Autodesk Inventor part; units mm, degrees
ref_plane "YZ Plane" through (0, 0, 0) normal (1, 0, 0) x (0, 1, 0)
ref_plane "XZ Plane" through (0, 0, 0) normal (0, 1, 0) x (-1, 0, 0)
ref_plane "XY Plane" through (0, 0, 0) normal (0, 0, 1) x (1, 0, 0)
sketch "Boceto1" plane through (0, 0, 0) normal (0, 0, 1) x (1, 0, 0)
  line L0 (-45, 21.0335) -> (-45, 0)
  line L1 (-43.1, 4) -> (-1.9, 4)
  line L2 (0, 0) -> (0, 15.6)
  line L3 (-4.7, 44) -> (-4.7, 21.3767)
  line L4 (-4.7, 44) -> (-9.9, 44)
  line L5 (-8.5, 42.6) -> (-6.1, 42.6)
  line L6 (-6.1, 36.1) -> (-8.5, 36.1)
  line L7 (-43.6, 19.6) -> (-5.4, 19.6)
  line L8 (-1.4, 15.6) -> (-1.4, 5.9)
  line L9 (-1.9, 5.4) -> (-43.1, 5.4)
  line L10 (-43.6, 5.9) -> (-43.6, 19.6)
  arc A0 (0, 15.6) -> (-4.3017, 20.8871) centre (-5.4, 15.6) ccw
  arc A1 (-1.4, 15.6) -> (-5.4, 19.6) centre (-5.4, 15.6) ccw
  line L11 (-1.4, 3.5) -> (-1.4, 1.7468)
  line L12 (-2.5, 0) -> (0, 0)
  line L13 (-6.1, 21.5) -> (-6.1, 34.7)
  line L14 (-6.1, 36.1) -> (-6.1, 42.6)
  line L15 (-43.6, 3.5) -> (-43.6, 1.6777)
  line L16 (-42.5, 0) -> (-45, 0)
  line L17 (-42.5, 0) -> (-42.5, 0.4554)
  line L18 (-2.5, 0) -> (-2.5, 0.7)
  line L19 (-43.6, 21) -> (-43.6, 24)
  line L20 (-42.48, 25.4) -> (-45, 25.4)
  line L21 (-45, 25.4) -> (-45, 21.0335)
  line L22 (-24, 21) -> (-24, 25.4)
  line L23 (-24, 25.4) -> (-26.39, 25.4)
  line L24 (-25.4, 24) -> (-25.4, 21)
  line L25 (-6.6, 21) -> (-24, 21)
  line L26 (-25.4, 21) -> (-43.6, 21)
  line L27 (-41.6, 24) -> (-43.6, 24)
  line L28 (-27.4, 24) -> (-25.4, 24)
  line L29 (-42.7447, 0.8853) -> (-43.3553, 1.2478)
  line L30 (-2.5, 0.7) -> (-1.6082, 1.3408)
  line L31 (-41.6, 24) -> (-41.6, 24.695)
  line L32 (-27.4, 24) -> (-27.4, 24.7058)
  line L33 (-42.48, 25.4) -> (-41.6, 24.695)
  line L34 (-27.4, 24.7058) -> (-26.39, 25.4)
  line L35 (-6.1, 34.7) -> (-9.9, 34.7)
  line L36 (-8.5, 37.35) -> (-8.5, 36.1)
  line L37 (-8.5, 41.35) -> (-8.5, 42.6)
  line L38 (-8.5, 37.35) -> (-9.2058, 37.35)
  line L39 (-8.5, 41.35) -> (-9.2058, 41.35)
  line L40 (-9.9, 44) -> (-9.9, 42.36)
  line L41 (-9.9, 42.36) -> (-9.2058, 41.35)
  line L42 (-9.9, 34.7) -> (-9.9, 36.34)
  line L43 (-9.9, 36.34) -> (-9.2058, 37.35)
  arc A2 (-6.6, 21) -> (-6.1, 21.5) centre (-6.6, 21.5) ccw
  arc A3 (-4.7, 21.3767) -> (-4.3017, 20.8871) centre (-4.2, 21.3767) ccw
  arc A4 (-1.9, 5.4) -> (-1.4, 5.9) centre (-1.9, 5.9) ccw
  arc A5 (-1.4, 3.5) -> (-1.9, 4) centre (-1.9, 3.5) ccw
  arc A6 (-1.6082, 1.3408) -> (-1.4, 1.7468) centre (-1.9, 1.7468) ccw
  arc A7 (-43.6, 5.9) -> (-43.1, 5.4) centre (-43.1, 5.9) ccw
  arc A8 (-43.1, 4) -> (-43.6, 3.5) centre (-43.1, 3.5) ccw
  arc A9 (-43.6, 1.6777) -> (-43.3553, 1.2478) centre (-43.1, 1.6777) ccw
  line L44 (0, 4) -> (0, 4.0335)
  arc A10 (-42.5, 0.4554) -> (-42.7447, 0.8853) centre (-43, 0.4554) ccw
  point P0 (-8.5, 41.975)
  point P1 (-42.5, 4)
  point P2 (-6.1, 39.35)
  point P3 (-42.5, 0.74)
  dimension "d16" = 5.4
  dimension "d17" = 4
  dimension "d32" = 1.4
  dimension "d35" = 1.4
  dimension "d37" = 3
  dimension "d38" = 25.4
  dimension "d44" = 18.2
  dimension "d50" = 0.7
  dimension "d53" = 40.3
  dimension "d54" = 37.5
  dimension "d55" = 1.4
  dimension "d57" = 17
  dimension "d62" = 30.7
  dimension "d63" = 35.7
  dimension "d64" = 4.4
  dimension "d66" = 3
  dimension "d69" = 4.4
  dimension "d71" = 3.4
  dimension "d72" = 3.4
  dimension "d73" = 0.88
  dimension "d74" = 1.01
  dimension "d75" = 34.5
  dimension "d76" = 38.7
  dimension "d77" = 0.695
  dimension "d78" = 0.7058
  dimension "d81" = 23
  dimension "d82" = 44
  dimension "d84" = 6.5
  dimension "d85" = 2.4
  dimension "d86" = 2.4
  dimension "d87" = 9.3
  dimension "d88" = 1.4
  dimension "d99" = 1.4
  dimension "d100" = 1.4
  dimension "d102" = 1.4
  dimension "d140" = 111
  dimension "d141" = 4
  dimension "d142" = 6.02
  dimension "d143" = 0.7058
  dimension "d144" = 0.7058
  dimension "d199" = 1.4
  dimension "d201" = 14.2
  dimension "d202" = 0.5
  dimension "d203" = 3.01
  dimension "d204" = 2
  dimension "d205" = 2.5
  dimension "d206" = 4.7
  dimension "d207" = 6.1
  dimension "d208" = 42.5
  dimension "d209" = 41.35
  dimension "d210" = 5.4
  dimension "d211" = 4
  dimension "d216" = 4.0335
  dimension "d218" = 0.74
  dimension "d219" = 0.5
  dimension "d220" = 45
  dimension "d221" = 5.2
  dimension "d225" = 1.4
extrude "Extrusión1" add sketch "Boceto1" against normal blind 2100
sketch "Boceto2" plane through (0, 0, 0) normal (1, 0, 0) x (0, 1, 0)
  line L0 (0, 0) -> (15.6, 0)
  line L1 (0, 0) -> (0, -2100)
  line L2 (15.6, -2100) -> (0, -2100)
  line L3 (15.6, 0) -> (15.6, -2100)
  line L4 (15.6, 0) -> (20.8871, 0)
  line L5 (15.6, 0) -> (15.6, -2100)
  line L6 (20.8871, -2100) -> (15.6, -2100)
  line L7 (20.8871, 0) -> (20.8871, -2100)
  line L8 (20.8871, 0) -> (21.3767, 0)
  line L9 (20.8871, 0) -> (20.8871, -2100)
  line L10 (21.3767, -2100) -> (20.8871, -2100)
  line L11 (21.3767, 0) -> (21.3767, -2100)
  line L12 (21.3767, 0) -> (44, 0)
  line L13 (21.3767, 0) -> (21.3767, -2100)
  line L14 (44, -2100) -> (21.3767, -2100)
  line L15 (44, 0) -> (44, -2100)
  line L16 (0, 0) -> (44, -44)
  line L17 (44, 0) -> (44, -44)
  line L18 (0, 0) -> (44, 0)
  dimension "d222" = 45
extrude "Extrusión2" cut sketch "Boceto2" against normal through all contours L0 L3 L16 | L4 L7 L16 L3 | L8 L11 L16 L7 | L12 L15 L16 L11
sketch "Boceto3" plane through (-43.1, 4, -2100) normal (0, -1, 0) x (1, 0, 0)
  circle A0 centre (19, 2054) radius 3
  line L0 (41.2, 2096) -> (0, 2096)
  line L1 (40.6, 2100) -> (40.6, 0)
  line L2 (0.6, 2100) -> (0.6, 0)
  point P0 (43.1, 2100)
  dimension "d227" = 6
  dimension "d228" = 42
  dimension "d229" = 21.6
  dimension "d230" = 18.4
hole "Agujero1" at (-24.1, 4, -46) direction (0, 1, 0) diameter 6 depth 1.4 countersink diameter 7 countersink angle 90
thread "Rosca1"
properties part number "SP40-01 MARCO BATIENTE - PAÑO FIJO 2100MM" material "Aluminio"
The model under review builds one solid part; all positions refer to its coordinate system, in mm. A direction names the side the tool comes from. Give positions to 0.01 mm unless a question says otherwise; leave off trailing zeros. Answer as a JSON object with one key per item and string values. Group by question number.
Q1. Tool access review of faces 3 (the flat face through (-25, 19.6, -1045)), 4 (the flat face through (-19, 20, -20)): name each direction out of +Z, -Z, +X, -X, +Y, -Y from which nothing blocks a thin tool from reaching the whole face with its end or side.
Q2. Insertion check: pin 1 (9 mm diameter, centred on x = -35.5, z = -1023, fed in from +Y); pin 2 (0.6 mm diameter, centred on x = -26, z = -873.5, fed in from -Y); pin 3 (1 mm diameter, centred on y = 35, z = -1822.5, fed in from -X). Each pin has a flat end and moves straight along its axis. Give the tip position at first contact, or say it passes through.
Q3. Draft analysis for pull direction X (two halves, no side actions). For faces 1 (the flat face through (-22, 5.4, -1038)), 2 (the flat face through (-21, 20, -2100)), state which applies: pulls with the +X half, pulls with the -X half, needs draft (parallel to the pull), parting line crosses it, or undercut.
Q4. Wall thickness on line 1 along Y through (x, z) = (-26, -969); line 2 along X through (y, z) = (23, -1306.5); line 3 along Y through (x, z) = (-42, -118.5): over which ranges is each line inside the solid? List them lowest first.
Answer below:
{
 "1": {"face 3": "+Z, -Z", "face 4": "+Z, +X, -X, +Y"},
 "2": {"pin 1": "stops at y = 21", "pin 2": "stops at y = 4", "pin 3": "stops at x = -9.9"},
 "3": {"face 1": "undercut", "face 2": "needs draft"},
 "4": {"line 1": "y = 4 to 5.4, 19.6 to 21, 24 to 25.4", "line 2": "x = -45 to -43.6, -25.4 to -24, -6.1 to -4.7", "line 3": "y = 4 to 5.4, 19.6 to 21, 24 to 25.02"}
}
